from build123d import *

# Parameters (mm, degrees)
F1_DEPTH    = 290
F2_T1_DEPTH = 611.1034588044
F3_R        = 4.25
F4_DEPTH    = 25
F5_W        = 60
F5_H        = 130.8605410159
F6_DEPTH    = 10.2
F7_R        = 5


# Not quite as in the source:
# - a fillet or chamfer that OpenCascade refuses, or shapes differently, is made with other operations: its cross-section is extruded or revolved along the edge and cut away or added
# - a pattern or mirror of a feature is missing from the dataset's text; its kind, count and spacing are read off the source's solid


with BuildPart() as f1:
    # F0 (on Right) → F1 (new body, symmetric)
    with BuildSketch(Plane.YZ):
        with BuildLine():
            ThreePointArc((-25.83, -74.2), (-25.2442135624, -75.6142135624), (-23.83, -76.2))
            Line((-23.83, -76.2), (23.83, -76.2))
            ThreePointArc((23.83, -76.2), (25.2442135624, -75.6142135624), (25.83, -74.2))
            Line((25.83, -74.2), (25.83, 74.2))
            ThreePointArc((25.83, 74.2), (25.2442135624, 75.6142135624), (23.83, 76.2))
            Line((23.83, 76.2), (-23.83, 76.2))
            ThreePointArc((-23.83, 76.2), (-25.2442135624, 75.6142135624), (-25.83, 74.2))
            Line((-25.83, 74.2), (-25.83, 69.4007524114))
            Line((-25.83, 69.4007524114), (13.2857787137, 65.978565209))
            ThreePointArc((13.2857787137, 65.978565209), (16.5363866841, 64.3755427566), (17.85, 60.9975917185))
            Line((17.85, 60.9975917185), (17.85, -60.9975917185))
            ThreePointArc((17.85, -60.9975917185), (16.5363866841, -64.3755427566), (13.2857787137, -65.978565209))
            Line((13.2857787137, -65.978565209), (-25.83, -69.4007524114))
            Line((-25.83, -69.4007524114), (-25.83, -74.2))
        make_face()
    extrude(amount=F1_DEPTH, both=True)

    # F2: fillet of radius 7 on 2 edges, made by hand

    # F2_s2 → F2_t1 (cut)
    with BuildSketch(Plane.YZ.offset(-305.5517294022)):
        with BuildLine():
            ThreePointArc((-25.83, -74.2), (-23.5930536317, -70.5297202282), (-19.6329798493, -68.8585834006))
            Line((-19.6329798493, -68.8585834006), (-19.6451816533, -68.7191161428))
            Line((-19.6451816533, -68.7191161428), (-25.842201804, -69.2612851537))
            Line((-25.842201804, -69.2612851537), (-25.97, -69.4007524114))
            ThreePointArc((-25.97, -69.4007524114), (-25.97, -71.8003762057), (-25.966142207, -74.1673610743))
            Line((-25.966142207, -74.1673610743), (-25.83, -74.2))
        make_face()
        with BuildLine():
            ThreePointArc((-19.6329798493, 68.8585834006), (-23.5930536317, 70.5297202282), (-25.83, 74.2))
            Line((-25.83, 74.2), (-25.966142207, 74.1673610743))
            ThreePointArc((-25.966142207, 74.1673610743), (-25.97, 71.8003762057), (-25.97, 69.4007524114))
            Line((-25.97, 69.4007524114), (-25.842201804, 69.2612851537))
            Line((-25.842201804, 69.2612851537), (-19.6451816533, 68.7191161428))
            Line((-19.6451816533, 68.7191161428), (-19.6329798493, 68.8585834006))
        make_face()
    extrude(amount=F2_T1_DEPTH, mode=Mode.SUBTRACT)

    # F3 (on face) → F4 (cut)
    with BuildSketch(Plane.XY.offset(76.2)):
        with Locations((-275, 0.83)):
            Circle(F3_R)
        with Locations((-165, 0.83)):
            Circle(F3_R)
        with Locations((-55, 0.83)):
            Circle(F3_R)
        with Locations((55, 0.83)):
            Circle(F3_R)
        with Locations((165, 0.83)):
            Circle(F3_R)
        with Locations((275, 0.83)):
            Circle(F3_R)
    extrude(amount=-F4_DEPTH, mode=Mode.SUBTRACT)

    # F5 (on face) → F6 (cut)
    with BuildSketch(Plane.XY.offset(76.2)):
        with Locations((-277.5, 8.7228175253)):
            Rectangle(F5_W, F5_H)
        with Locations((277.5, 8.7228175253)):
            Rectangle(F5_W, F5_H)
    f6 = extrude(amount=-F6_DEPTH, mode=Mode.SUBTRACT)

    # F6_copies: F6 across plane
    add(f6.mirror(Plane(origin=(0, 0, 0), x_dir=(-1, 0, 0), z_dir=(0, 0, -1))), mode=Mode.SUBTRACT)

    # F7
    f7_edges = [f1.edges().sort_by_distance(p)[0] for p in [
        (-290, 19.435389, 66),
        (290, 19.435389, 66),
        (290, 19.435389, -66),
        (-290, 19.435389, -66),
    ]]
    fillet(f7_edges, radius=F7_R)


solid = f1.part
Part model, mm, in its own coordinate system. A direction names the side the tool comes from. Round coordinates to 2 decimals unless told otherwise and drop trailing zeros. Loops run counter-clockwise (first coordinate to the right, second up) from the corner with the lowest first, then second, coordinate; pieces in that order, holes last. Notation, with made-up numbers: (60.25, 56.5) - (85.25, 56.5) arc R16 ccw to (85.25, 65.5) - close; hole circle Ø6 at (61, -12.5). An arc over 180 degrees is marked (long way). Answer as a JSON object with one key per item and string values.
Item 1: Band-saw the part on B-B on z = -45. List the corners of the cut face in (x, y).
Output:
{"outline": "(-290, 17.85) - (290, 17.85) - (290, 25.83) - (-290, 25.83) - close"}
Item 2: Wall check: L1, parallel to X at y = 0, z = 72; L2, parallel to Z at x = 206.5, y = -20; L3, parallel to Y at x = -198.5, z = -6. Give the ranges that are in metal, low to high.
Output:
{"L1": "-247.5 to -169.17, -160.83 to -59.17, -50.83 to 50.83, 59.17 to 160.83, 169.17 to 247.5", "L2": "-76.2 to -68.9, 68.9 to 76.2", "L3": "17.85 to 25.83"}
Item 3: Band-saw the part on A-A on x = -218.5. List the corners of the cut face in (y, z).
Output:
{"outline": "(-25.83, -74.2) arc R2 ccw to (-23.83, -76.2) - (23.83, -76.2) arc R2 ccw to (25.83, -74.2) - (25.83, 74.2) arc R2 ccw to (23.83, 76.2) - (-23.83, 76.2) arc R2 ccw to (-25.83, 74.2) arc R7 ccw to (-19.63, 68.86) - (13.29, 65.98) arc R5 cw to (17.85, 61) - (17.85, -61) arc R5 cw to (13.29, -65.98) - (-19.63, -68.86) arc R7 ccw to start"}
Item 4: Pin check, flat tips, straight feed: pin 1 (4 mm diameter, centred on x = 264, y = 21, fed in from +Z); pin 2 (8 mm diameter, centred on y = -8, z = -69, fed in from +X); pin 3 (5 mm diameter, centred on x = -208.5, z = -9.5, fed in from -Y). Stop position of each tip, or through.
Output:
{"pin 1": "z = 66", "pin 2": "x = 247.5", "pin 3": "y = 17.85"}
Item 5: Tool access for faces 4 (the face through (247.5, 0, -72)), 5 (the face through (-267, 20, 66)), 6 (the face through (4, 17.85, 1)): list every direction of +Z, -Z, +X, -X, +Y, -Y with a clear straight run to the whole face (end or side of a thin tool).
Output:
{"face 4": "-Z, +X, +Y, -Y", "face 5": "+Z, -X, +Y, -Y", "face 6": "+X, -X, -Y"}
Item 6: Pull direction Z, two halves, no side cores. Call faces 1 (the face through (4, -2.94, -67.4)), 2 (the face through (-267, 20, -66)), 3 (the face through (4, 25.83, -1)): pulls with the +Z half, pulls with the -Z half, needs draft (parallel to the pull), parting line crosses it, or undercut.
Output:
{"face 1": "undercut", "face 2": "pulls with the -Z half", "face 3": "needs draft"}
